Design review of the part built by this model. Coordinates are the model's own, in mm. A direction names the side the tool comes from. Coordinates: 2 decimals unless noted, no trailing zeros. Loops run counter-clockwise (first coordinate to the right, second up) from the corner with the lowest first, then second, coordinate; pieces in that order, holes last.
Autodesk Fusion 360 part; units mm, degrees
sketch "Esquisse1" plane through (0, 0, 0) normal (0, 0, 1) x (1, 0, 0)
  line L0 (-57.5, 20) -> (57.5, 20)
  line L1 (57.5, 20) -> (57.5, -20)
  line L2 (57.5, -20) -> (-57.5, -20)
  line L3 (-57.5, -20) -> (-57.5, 20)
  line L4 (0, 1.75) -> (0, 22.5)
  line L5 (1.75, 0) -> (22.5, 0)
  dimension "d1" = 115
  dimension "d2" = 40
extrude "Extrusion1" add sketch "Esquisse1" along normal blind 30
sketch "Esquisse2" plane through (0, 0, 30) normal (0, 0, 1) x (-1, 0, 0)
  line L0 (57.5, 20) -> (-57.5, 20)
  line L1 (-57.5, 20) -> (-57.5, -20)
  line L2 (-57.5, -20) -> (57.5, -20)
  line L3 (57.5, -20) -> (57.5, 20)
  circle A0 centre (40, 0) radius 7.625
  line L4 (0, -1.75) -> (0, -22.5)
  line L5 (-1.75, 0) -> (-22.5, 0)
  dimension "d5" = 15.25
  dimension "d6" = 40
extrude "Extrusion2" cut sketch "Esquisse2" against normal blind 25 contours A0
mirror "Symétrie miroir1" about plane through (0, 0, 0) normal (1, 0, 0) of "Extrusion2"
sketch "Esquisse3" plane through (0, 0, 30) normal (0, 0, 1) x (-1, 0, 0)
  circle A0 centre (-40, 0) radius 7.625
  circle A1 centre (40, 0) radius 7.625
  line L0 (57.5, 20) -> (-57.5, 20)
  line L1 (-57.5, 20) -> (-57.5, -20)
  line L2 (-57.5, -20) -> (57.5, -20)
  line L3 (57.5, -20) -> (57.5, 20)
sketch "Esquisse4" plane through (0, 0, 30) normal (0, 0, 1) x (1, 0, 0)
  circle A0 centre (-40, 0) radius 12 construction
  line L0 (1.75, 0) -> (22.5, 0)
  point P0 (-52, 0)
  dimension "d11" = 24
  dimension "d12" = 40
sketch "Esquisse5" plane through (0, 0, 30) normal (0, 0, 1) x (1, 0, 0)
  circle A0 centre (0, 0) radius 5.15
  dimension "d20" = 10.3
extrude "Extrusion3" cut sketch "Esquisse5" against normal blind 75
sketch "Esquisse6" plane through (0, 0, 30) normal (0, 0, 1) x (1, 0, 0)
  point P0 (-8, 0)
  dimension "d23" = 8
hole "Perçage2" at (-8, 0, 30) direction (0, 0, -1) diameter 4.5 depth 50 tip angle 118
pattern_circular "Réseau C2" count 4 over 360 about axis through (0, 0, 30) along (0, 0, -1) of "Perçage2"
sketch "Esquisse7" plane through (0, 0, 30) normal (0, 0, 1) x (1, 0, 0)
sketch "Esquisse8" plane through (0, 0, 30) normal (0, 0, 1) x (-1, 0, 0)
  circle A0 centre (40, 0) radius 5
  dimension "d31" = 10
extrude "Extrusion4" cut sketch "Esquisse8" against normal blind 51
mirror "Symétrie miroir4" about plane through (0, 0, 0) normal (1, 0, 0) of "Extrusion4"
sketch "Esquisse9" plane through (0, 0, 0) normal (0, 0, 1) x (1, 0, 0)
  circle A0 centre (-40, 0) radius 10
  dimension "d36" = 20
extrude "Extrusion5" add sketch "Esquisse9" against normal blind 25
sketch "Esquisse10" plane through (0, 0, -25) normal (0, 0, -1) x (1, 0, 0)
  circle A0 centre (-40, 0) radius 10
sketch "Esquisse11" plane through (0, 0, -25) normal (0, 0, -1) x (1, 0, 0)
  circle A0 centre (-40, 0) radius 7.625
  dimension "d39" = 15.25
extrude "Extrusion6" cut sketch "Esquisse11" against normal blind 25
mirror "Symétrie miroir5" about plane through (0, 0, 0) normal (1, 0, 0) of "Extrusion6", "Extrusion5"
sketch "Esquisse12" plane through (0, 20, 0) normal (0, 1, 0) x (-1, 0, 0)
  line L0 (-57.5, 0) -> (57.5, 0)
  line L1 (57.5, 0) -> (57.5, 30)
  line L2 (57.5, 30) -> (-57.5, 30)
  line L3 (-57.5, 30) -> (-57.5, 0)
  circle A0 centre (0, 15) radius 6
  dimension "d44" = 12
extrude "Extrusion7" cut sketch "Esquisse12" against normal blind 4 contours A0
sketch "Esquisse13" plane through (0, 20, 0) normal (0, 1, 0) x (-1, 0, 0)
  circle A0 centre (0, 15) radius 6
  line L0 (-57.5, 0) -> (57.5, 0)
  line L1 (57.5, 0) -> (57.5, 30)
  line L2 (57.5, 30) -> (-57.5, 30)
  line L3 (-57.5, 30) -> (-57.5, 0)
sketch "Esquisse14" plane through (0, 20, 0) normal (0, 1, 0) x (-1, 0, 0)
  line L0 (57.5, 0) -> (-57.5, 0)
  point P0 (12, 15)
  point P1 (0, 15)
  dimension "d47" = 12
  dimension "d48" = 15
hole "Perçage3" at (-12, 20, 15) direction (0, -1, 0) diameter 2.6 depth 16 tip angle 118
mirror "Symétrie miroir6" about plane through (0, 0, 0) normal (1, 0, 0) of "Perçage3"
sketch "Esquisse15" plane through (-57.5, 0, 0) normal (-1, 0, 0) x (0, -1, 0)
  line L0 (-20, 0) -> (20, 0)
  line L1 (20, 0) -> (20, 30)
  line L2 (20, 30) -> (-20, 30)
  line L3 (-20, 30) -> (-20, 0)
  circle A0 centre (0, 15) radius 6
  line L4 (20, 0) -> (-20, 0)
  dimension "d54" = 12
  dimension "d55" = 15
  dimension "d56" = 20
extrude "Extrusion8" cut sketch "Esquisse15" against normal blind 5 contours A0
sketch "Esquisse16" plane through (-57.5, 0, 0) normal (-1, 0, 0) x (0, -1, 0)
  circle A0 centre (0, 15) radius 6
  line L0 (-20, 0) -> (20, 0)
  line L1 (20, 0) -> (20, 30)
  line L2 (20, 30) -> (-20, 30)
  line L3 (-20, 30) -> (-20, 0)
  line L4 (20, 0) -> (-20, 0)
  point P0 (12, 15)
  dimension "d59" = 12
  dimension "d60" = 15
hole "Perçage4" at (-57.5, -12, 15) direction (1, 0, 0) diameter 2.6 depth 16 tip angle 118
mirror "Symétrie miroir7" about plane through (0, 0, 0) normal (0, 1, 0) of "Perçage4"
mirror "Symétrie miroir8" about plane through (0, 0, 0) normal (1, 0, 0) of "Symétrie miroir7", "Perçage4", "Extrusion8"
equation "d23 = ( 19.5 / 2 ) * 1 mm - ( 3.5 / 2 ) * 1 mm"
Q1. Take a section at D-D, the plane y = 0. Give the number of separate pieces and of enclosed holes in the cut face, then the cut area to 3 significant figures.
Q2. The part is to be moulded in two halves that separate along Z. For faces 6 (the flat face through (-57.5, -0.3, 21.5)), 7 (the conical face through (40.855, 12.2, 15.104)), 8 (the flat face through (-47, -4, -25)), 9 (the conical face through (11.78, 3.355, 14.951)), say which applies: pulls with the +Z half, pulls with the -Z half, needs draft (parallel to the pull), parting line crosses it, or undercut.
Q3. For line 1 (Y direction, x = 0, z = 18.5); line 2 (Y direction, x = 0, z = 2); line 3 (Y direction, x = 40, z = 24.25) (3 decimals), list the stretches that pass through material, from the lowest coordinate up.
Q4. Clearance check with flat-ended pins moving along their axes: pin 1 Ø7 at (y, z) = (0, 15) entering from +X; pin 2 Ø5 at (x, y) = (24, 8) entering from -Z; pin 3 Ø3.5 at (x, z) = (1.5, 15) entering from +Y. State where each tip first meets the part, or that it passes through.
Q5. Take a section at A-A, the plane z = 1.5. Write out the cut boundary in (x, y).
Q6. Machinability: for faces 1 (the cylindrical face through (49.39, -10.71, 14.83)), 2 (the cylindrical face through (-47.618, -0.335, -12.675)), 3 (the flat face through (38, 5, 5)), 4 (the cylindrical face through (-13.29, 11.89, 14.83)), 5 (the cylindrical face through (-49.39, 10.71, 14.83)), which of the approach directions +Z, -Z, +X, -X, +Y, -Y give a long, thin tool a straight path to every point of the face, cutting with its end or side? Answer none if there is none.
Q7. Take a section at C-C, the plane y = -16. Write out the cut boundary in (x, z).
Q8. Take a section at B-B, the plane x = 8. Write out the cut boundary in (y, z), then the cut area to 4 significant figures.
Entries:
1. separate pieces: 5
1. enclosed holes: 0
1. area: 2,510 mm2
2. face 6: needs draft
2. face 7: undercut
2. face 8: pulls with the -Z half
2. face 9: undercut
3. line 1: y = -20 to -10.25, -5.75 to -5.15, 5.15 to 5.75, 10.25 to 16
3. line 2: y = -20 to -10.25, -5.75 to -5.15, 5.15 to 5.75, 10.25 to 20
3. line 3: y = -20 to -7.625, 7.625 to 20
4. pin 1: stops at x = 52.5
4. pin 2: stops at z = 0
4. pin 3: stops at y = 16
5. outline: (-57.5, -20) - (57.5, -20) - (57.5, 20) - (-57.5, 20) - close; hole circle Ø10 at (-40, 0); hole circle Ø4.5 at (-8, 0); hole circle Ø10.3 at (0, 0); hole circle Ø4.5 at (0, -8); hole circle Ø4.5 at (0, 8); hole circle Ø4.5 at (8, 0); hole circle Ø10 at (40, 0)
6. face 1: +X
6. face 2: -Z
6. face 3: +Z
6. face 4: +Y
6. face 5: -X
7. outline: (-57.5, 0) - (57.5, 0) - (57.5, 30) - (-57.5, 30) - close
8. outline: (-20, 0) - (-2.25, 0) - (-2.25, 30) - (-20, 30) - close; (2.25, 0) - (20, 0) - (20, 30) - (2.25, 30) - close
8. area: 1,065 mm2
